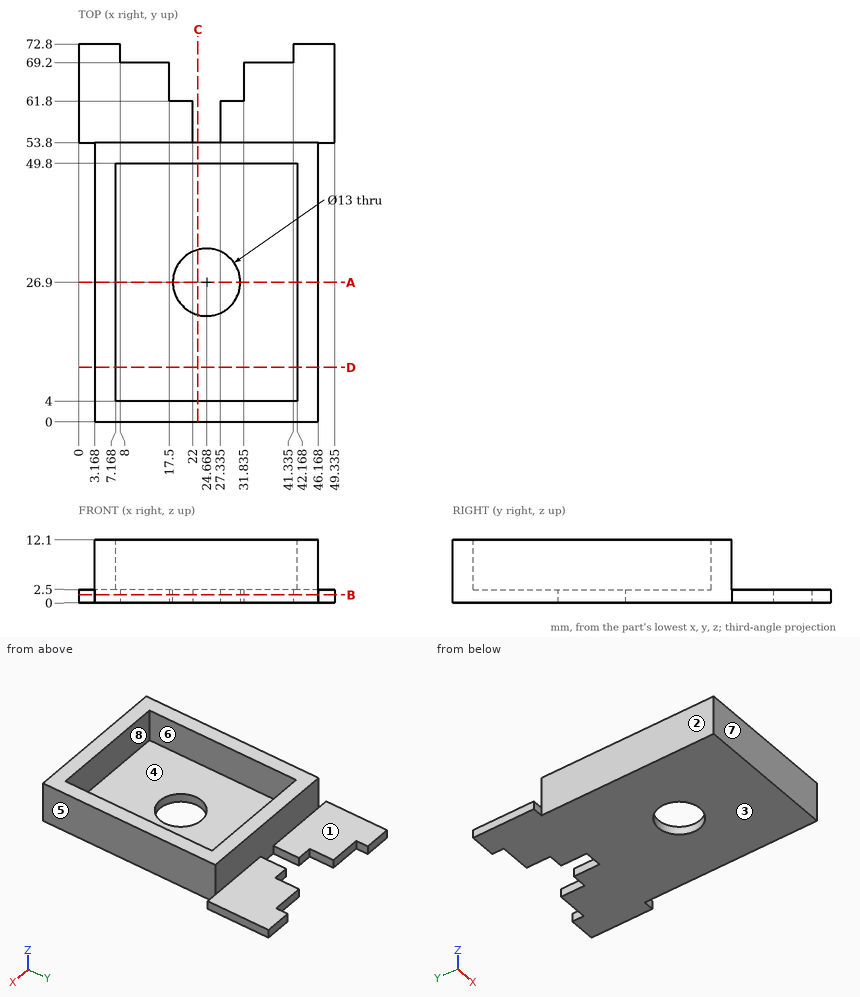
Geometry check sheet. Reference: drawing and pictorial views, mm from the part's lowest x, y, z. A direction names the side the tool comes from. Coordinates: 2 decimals unless noted, no trailing zeros. Write each loop counter-clockwise with the first axis right and the second up, starting at its lowest first coordinate (ties: lowest second). Pieces come first, ordered by that corner, then holes. Notation, with made-up numbers: M -38,26 L 9,26 A34 ccw 9,63 Z; hole C 77.25,4 d6. An arc over 180 degrees is marked long. One line per question, with ' | ' between items.
1) Sectioned sample at B-B on z = 1.5. Record the cut outline in (x, y) (1 decimal).
Solutions:
outline: M 0,53.8 L 3.2,53.8 L 3.2,0 L 46.2,0 L 46.2,53.8 L 49.3,53.8 L 49.3,72.8 L 41.3,72.8 L 41.3,69.2 L 31.8,69.2 L 31.8,61.8 L 27.3,61.8 L 27.3,53.8 L 22,53.8 L 22,61.8 L 17.5,61.8 L 17.5,69.2 L 8,69.2 L 8,72.8 L 0,72.8 Z; hole C 24.7,26.9 d13
2) Sectioned sample at C-C on x = 23. Record the cut outline in (y, z), then the cut area to 3 significant figures.
Solutions:
outline: M 0,0 L 20.62,0 L 20.62,2.5 L 4,2.5 L 4,12.1 L 0,12.1 Z; M 33.18,0 L 53.8,0 L 53.8,12.1 L 49.8,12.1 L 49.8,2.5 L 33.18,2.5 Z | area: 180 mm^2
3) Sectioned sample at D-D on y = 10.5. Record the cut outline in (x, z), then the cut area to 3 significant figures.
Solutions:
outline: M 3.17,0 L 46.17,0 L 46.17,12.1 L 42.17,12.1 L 42.17,2.5 L 7.17,2.5 L 7.17,12.1 L 3.17,12.1 Z | area: 184 mm^2
4) Access from +Z, -Z, +X, -X, +Y, -Y to the whole of each face (thin tool, end or side, straight path). Record for the marked faces 1, 2, 3 and 4.
Solutions:
face 1: +Z, +X, -X, +Y | face 2: +Z, -Z, -X, -Y | face 3: -Z, +X, -X, +Y, -Y | face 4: +Z
5) Sectioned sample at A-A on y = 26.9. Record the cut outline in (x, z).
Solutions:
outline: M 3.17,0 L 18.17,0 L 18.17,2.5 L 7.17,2.5 L 7.17,12.1 L 3.17,12.1 Z; M 31.17,0 L 46.17,0 L 46.17,12.1 L 42.17,12.1 L 42.17,2.5 L 31.17,2.5 Z
6) Release check for a two-part mould opening along X. For the marked faces 5, 6, 7 and 8 record: +X half, -X half, draft (parallel to the pull), parting line (faces both ways), or undercut.
Solutions:
face 5: +X half | face 6: undercut | face 7: draft | face 8: undercut
7) Material ranges on L1, parallel to X at y = 15, z = 6.75; L2, parallel to Y at x = 42, z = 6.25; L3, parallel to Z at x = 40.5, y = 37.5, recorded low to high.
Solutions:
L1: 3.17 to 7.17, 42.17 to 46.17 | L2: 0 to 4, 49.8 to 53.8 | L3: 0 to 2.5
8) Depth check by flat-ended pin: pin 1 Ø3.5 at (y, z) = (35, 7) entering from -X; pin 2 Ø3 at (x, y) = (12.5, 57.5) entering from +Z; pin 3 Ø0.8 at (x, z) = (35, 1.5) entering from +Y; pin 4 Ø8 at (x, y) = (24.67, 26.9) entering from -Z. Enter the tip coordinate at first touch or a pass-through.
Solutions:
pin 1: x = 3.17 | pin 2: z = 2.5 | pin 3: y = 69.2 | pin 4: through
